The model under review builds one solid part; all positions refer to its coordinate system, in mm. A direction names the side the tool comes from. Coordinates: 2 decimals unless noted, no trailing zeros. Order: outer loops, then holes, each group sorted by start corner. A loop starts at its lowest first (then second) coordinate and runs counter-clockwise, first axis right, second up. Notation, with made-up numbers: (17, -22) -> (45, -22) arc R26 cw to (45, -2) -> close; hole circle Ø7 at (59, 19.25). An arc over 180 degrees is marked (long way). Use one line per item in the form item = value. Start each with the question number.
(1) Mouldability with a two-part tool opening along Y and no side actions: class faces 1 (the cylindrical face through (-2.79, 20.16, 9.86)), 2 (the cylindrical face through (16.94, -2.52, 9.86)), 3 (the flat face through (8.839, 24, 10)), 4 (the cylindrical face through (9.18, 19.88, 9.86)) as +Y half, -Y half, draft (parallel to the pull), parting line (faces both ways), or undercut.
(2) Take a section at B-B (y = 17.5). State the section outline as (x, z) points, then the cut area to 3 significant figures.
(3) For faces 5 (the flat face through (-12.19, -21.7, 9.86)), 6 (the cylindrical face through (1.119, -23.462, 9.86)), 7 (the flat face through (-18.056, 13.302, 9.86)), 8 (the cylindrical face through (0.092, 39.79, 3.918)), list the 3-axis set-ups (+Z, -Z, +X, -X, +Y, -Y) from which the entire face can be reached by the end or side of a thin tool; tool diameter is ignored.
(4) Take a section at D-D (y = 0.5). State the section outline as (x, z) points.
(5) Take a section at C-C (z = 17.5). State the section outline as (x, y) points.
(6) Insertion check: pin 1 Ø3 at (x, z) = (9.5, 12) entering from +Y; pin 2 Ø4 at (y, z) = (-18.5, 8.5) entering from +X; pin 3 Ø1.3 at (y, z) = (23.5, 8) entering from -X; pin 4 Ø5 at (x, y) = (-3.5, 24) entering from +Z. Each pin has a flat end and moves straight along its axis. Give the tip position at first contact, or say it passes through.
(7) Wall thickness on line 1 along Y through (x, z) = (-12.5, 18.75); line 2 along Y through (x, z) = (-9.5, 8.5); line 3 along X through (y, z) = (-21.5, 10.25): over which ranges is each line inside the solid? List them lowest first.
```python
from build123d import *

# Parameters (mm, degrees)
F1_DEPTH      = 20
F4_END_RADIUS = 18.58687693
F3_W          = 20.205357112
F3_H          = 20.0386047363
F4_REACH      = 81.284821593
F5_R          = 1
F6_R          = 5
F7_R          = 1
F8_R          = 6.25
F9_DEPTH      = 30


# Not quite as in the source:
# - a feature of the source that left no trace in its solid (it failed there, or was rolled back) is left out


with BuildPart() as f1:
    # F0 (on Top) → F1 (new body)
    with BuildSketch(Plane.XY):
        with BuildLine():
            ThreePointArc((-16.300464081, 12.3786436003), (-3.0365664125, 20.1688822052), (9.8326279785, 11.7425760982))
            ThreePointArc((9.8326279785, 11.7425760982), (12.939174946, -2.2913182786), (9.8326279785, -16.3252126554))
            ThreePointArc((9.8326279785, -16.3252126554), (0.5036385974, -23.5957971339), (-10.8497184243, -20.2802691412))
            Line((-10.8497184243, -20.2802691412), (-13.5972941331, -23.1872998815))
            ThreePointArc((-13.5972941331, -23.1872998815), (1.2549394728, -27.5246070039), (13.4589359939, -18.0133744302))
            ThreePointArc((13.4589359939, -18.0133744302), (16.939174946, -2.2913182786), (13.4589359939, 13.430737873))
            ThreePointArc((13.4589359939, 13.430737873), (-2.9392370682, 24.1676979047), (-19.8403485782, 14.2412272216))
            Line((-19.8403485782, 14.2412272216), (-16.300464081, 12.3786436003))
        make_face()
    extrude(amount=F1_DEPTH)

    f4_end = (Plane(origin=(-3.391499204, 5.5863240865, 10), x_dir=(-1, 0, 0), z_dir=(0, 0, -1)) * Cylinder(F4_END_RADIUS, 296.0871828679, mode=Mode.PRIVATE)).faces().sort_by_distance((-2.9392370682, 24.1676979047, 10))[0]
    # F3 (on offset) → F4 (join, up to the whole of a round face its end follows)
    with BuildSketch(Plane.XZ.offset(-25)):
        with Locations((-1.2632482685, 10.0193023682)):
            Rectangle(F3_W, F3_H)
    f4_long = extrude(amount=F4_REACH, mode=Mode.PRIVATE)
    add(split(f4_long, bisect_by=f4_end, keep=Keep.ALL, mode=Mode.PRIVATE).solids().sort_by_distance((-1.2632482685, 25, 10.0193023682))[0])

    # F5
    f5_edges = [f1.edges().sort_by_distance(p)[0] for p in [
        (-16.300464, 12.378644, 10),
        (-19.840349, 14.241227, 10),
        (-10.849718, -20.280269, 10),
        (-13.597294, -23.1873, 10),
    ]]
    fillet(f5_edges, radius=F5_R)

    # F6
    f6_edges = [f1.edges().sort_by_distance(p)[0] for p in [
        (8.83943, 19.581908, 10),
    ]]
    fillet(f6_edges, radius=F6_R)

    # F7
    f7_edges = [f1.edges().sort_by_distance(p)[0] for p in [
        (-11.365927, 22.375621, 10),
    ]]
    fillet(f7_edges, radius=F7_R)

    # F8 (on face) → F9 (join)
    with BuildSketch(Plane(origin=(0, 25, 0), x_dir=(-1, 0, 0), z_dir=(0, 1, 0))):
        with Locations((1.2632482685, 10.0193023682)):
            Circle(F8_R)
    extrude(amount=F9_DEPTH)


solid = f1.part
```
Findings:
q1.face_1 = undercut
q1.face_2 = parting line
q1.face_3 = draft
q1.face_4 = +Y half
q2.outline = (-17.66, 0) -> (-11.81, 0) -> (-11.81, 20) -> (-17.66, 20) -> close; (5.03, 0) -> (10.88, 0) -> (10.88, 20) -> (5.03, 20) -> close
q2.area = 234 mm²
q3.face_5 = +Z, -Z, -X
q3.face_6 = +Z, -Z
q3.face_7 = +Z, -Z, -X, -Y
q3.face_8 = +Y
q4.outline = (12.82, 0) -> (16.83, 0) -> (16.83, 20) -> (12.82, 20) -> close
q5.outline = (-19.32, 15.16) arc R1 ccw to (-18.93, 13.76) -> (-17.16, 12.83) arc R1 ccw to (-15.84, 13.19) arc R14.59 cw to (9.83, 11.74) arc R33.25 cw to (9.83, -16.33) arc R12.98 cw to (-10.15, -20.89) arc R1 ccw to (-11.51, -20.98) -> (-12.89, -22.44) arc R1 ccw to (-12.8, -23.89) arc R16.98 ccw to (13.46, -18.01) arc R37.25 ccw to (13.46, 13.43) arc R18.59 ccw to (10.19, 18.28) arc R5 cw to (8.84, 21.69) -> (8.84, 25) -> (-11.37, 25) -> (-11.37, 23) arc R1 cw to (-11.91, 22.11) arc R18.59 ccw to start
q6.pin_1 = 25
q6.pin_2 = 14.12
q6.pin_3 = -11.38
q6.pin_4 = 20.04
q7.line_1 = -24.14 to -22.03, 16.98 to 21.79
q7.line_2 = -26.05 to -21.39, 18.83 to 25
q7.line_3 = -12 to -9.35, 5.48 to 11.29
